Geometry check sheet. Reference: the model listing, model coordinates, mm. Coordinates: 2 decimals unless noted, no trailing zeros. Write each loop counter-clockwise with the first axis right and the second up, starting at its lowest first coordinate (ties: lowest second). Pieces come first, ordered by that corner, then holes. Notation, with made-up numbers: (45, 51.25) -> (97, 51.25) arc R17 cw to (97, 73.25) -> close; hole circle Ø8 at (35.25, 6.25). An arc over 180 degrees is marked (long way). One line per question, with ' | ' between items.
```python
from build123d import *


with BuildPart() as part:
    # Sketch1 → Revolve1 (revolve)
    with BuildSketch(Plane.XY, mode=Mode.PRIVATE) as revolve1_sk:
        with BuildLine():
            Line((2.805064434, 27.94), (1.905, 27.94))
            ThreePointArc((1.905, 27.94), (0, 27.305), (-1.905, 27.94))
            Line((-1.905, 27.94), (-2.805064434, 27.94))
            Line((-2.805064434, 27.94), (-2.805064434, 22.987))
            ThreePointArc((-2.805064434, 22.987), (-2.61907724, 22.537987194), (-2.170064434, 22.352))
            Line((-2.170064434, 22.352), (2.170064434, 22.352))
            ThreePointArc((2.170064434, 22.352), (2.61907724, 22.537987194), (2.805064434, 22.987))
            Line((2.805064434, 22.987), (2.805064434, 27.94))
        make_face()
    revolve(revolve1_sk.sketch.rotate(Axis((-23.195066381, 0, 0), (1, 0, 0)), 90), axis=Axis((-23.195066381, 0, 0), (1, 0, 0)))


solid = part.part
```
(1) Cross-section at C-C (x = -0.35). Record the cut outline in (y, z).
Answers below:
outline: circle Ø54.65 at (0, 0); hole circle Ø44.7 at (0, 0)
(2) Material ranges on line 1 (Z direction, x = -0.4, y = 17); line 2 (Y direction, x = 0.45, z = 0); line 3 (Y direction, x = -0.25, z = 9), recorded low to high.
Answers below:
line 1: z = -21.4 to -14.51, 14.51 to 21.4 | line 2: y = -27.34 to -22.35, 22.35 to 27.34 | line 3: y = -25.79 to -20.46, 20.46 to 25.79
(3) Draft check along Z on faces 1 (the face through (2.35, -27.7, -3.64)), 2 (the face through (-2.805, 23, 4)), 3 (the face through (0.03, 13.6, -17.74)). Enter one of: pulls with the +Z half, pulls with the -Z half, needs draft (parallel to the pull), parting line crosses it, or undercut.
Answers below:
face 1: parting line crosses it | face 2: needs draft | face 3: undercut
(4) Depth check by flat-ended pin: P1, Ø2, axis at x = 2, z = 12.5, coming from the -Y side. Enter the tip coordinate at first touch or a pass-through.
Answers below:
P1: stops at y = -25.46
(5) Cross-section at A-A (y = 0). Record the cut outline in (x, z) (3 decimals).
Answers below:
outline: (-2.805, -27.94) -> (-1.905, -27.94) arc R3.175 cw to (1.905, -27.94) -> (2.805, -27.94) -> (2.805, -22.987) arc R0.635 ccw to (2.17, -22.352) -> (-2.17, -22.352) arc R0.635 ccw to (-2.805, -22.987) -> close; (-2.805, 22.987) arc R0.635 ccw to (-2.17, 22.352) -> (2.17, 22.352) arc R0.635 ccw to (2.805, 22.987) -> (2.805, 27.94) -> (1.905, 27.94) arc R3.175 cw to (-1.905, 27.94) -> (-2.805, 27.94) -> close
